Drawing for the job (mm, zero at the part's lowest x, y, z). Give positions to 0.01 mm unless a question says otherwise; leave off trailing zeros. Write each loop counter-clockwise with the first axis right and the second up, starting at its lowest first coordinate (ties: lowest second). Pieces come first, ordered by that corner, then holes.
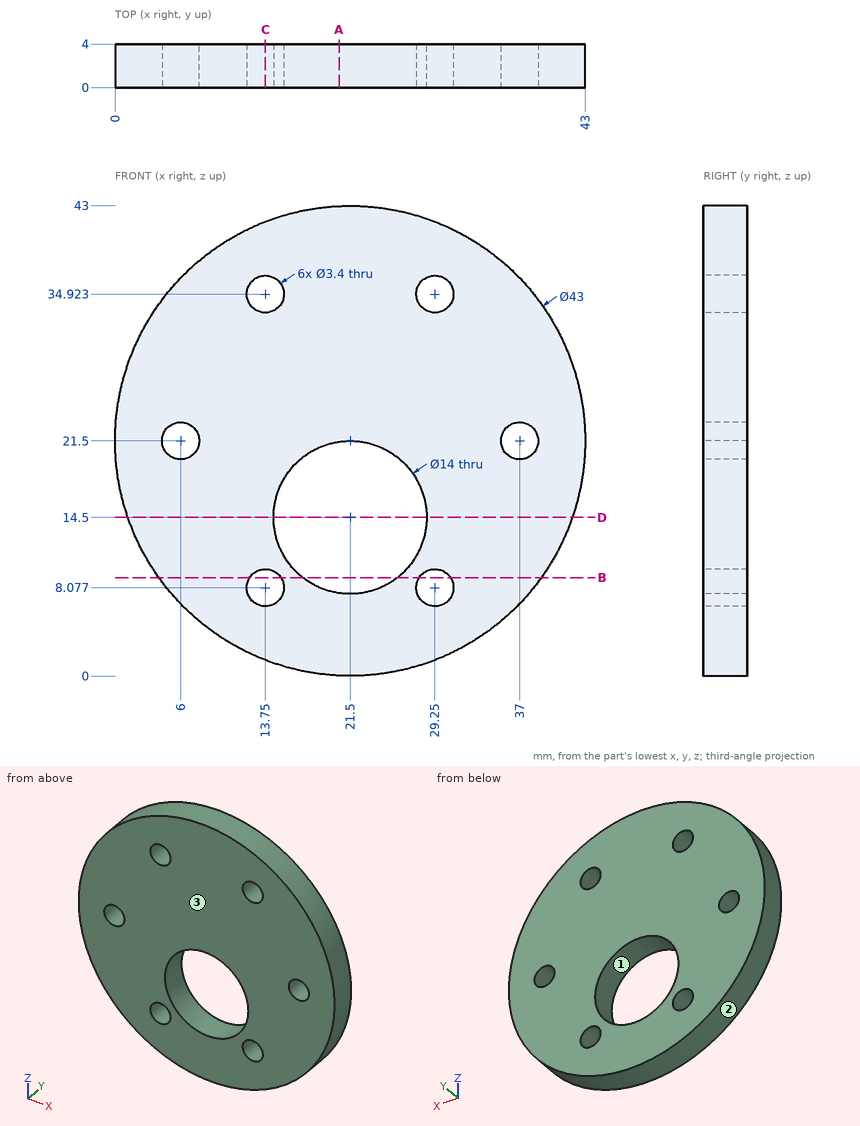
1. Pull direction X, two halves, no side cores. Call the marked faces 1, 2 and 3: +X half, -X half, draft (parallel to the pull), parting line (faces both ways), or undercut.
Calculated:
face 1: undercut
face 2: parting line
face 3: draft
2. Probe probe 1 along X at (y, z) = (2.4, 20.5) (1 decimal); probe 2 along Z at (x, y) = (21.5, 3.05); probe 3 along Z at (x, y) = (13.75, 2.45) (1 decimal). List the from-to ranges inside material, lowest first.
Calculated:
probe 1: x = 0 to 4.6, 7.4 to 17.9, 25.1 to 35.6, 38.4 to 43
probe 2: z = 0 to 7.5, 21.5 to 43
probe 3: z = 1.4 to 6.4, 9.8 to 33.2, 36.6 to 41.6
3. Slice it at A-A, the plane x = 20.5. Write the cut outline in (y, z), and give its area (3 significant figures).
Calculated:
outline: (0, 0.02) - (4, 0.02) - (4, 7.57) - (0, 7.57) - close; (0, 21.43) - (4, 21.43) - (4, 42.98) - (0, 42.98) - close
area: 116 mm2
4. Slice it at C-C, the plane x = 13.75. Write the cut outline in (y, z) (1 decimal).
Calculated:
outline: (0, 1.4) - (4, 1.4) - (4, 6.4) - (0, 6.4) - close; (0, 9.8) - (4, 9.8) - (4, 33.2) - (0, 33.2) - close; (0, 36.6) - (4, 36.6) - (4, 41.6) - (0, 41.6) - close
5. Pin check, flat tips, straight feed: P1, Ø4, axis at x = 6, z = 21.5, coming from the -Y side; P2, Ø3, axis at x = 13.75, z = 8.08, coming from the +Y side; P3, Ø2, axis at x = 11, y = 2.5, coming from the -Z side; P4, Ø2, axis at x = 31, y = 0.5, coming from the -Z side. Stop position of each tip, or through.
Calculated:
P1: stops at y = 0
P2: passes through
P3: stops at z = 2.21
P4: stops at z = 1.75
6. Slice it at B-B, the plane z = 9. Write the cut outline in (x, y).
Calculated:
outline: (4.01, 0) - (12.32, 0) - (12.32, 4) - (4.01, 4) - close; (15.18, 0) - (17.17, 0) - (17.17, 4) - (15.18, 4) - close; (25.83, 0) - (27.82, 0) - (27.82, 4) - (25.83, 4) - close; (30.68, 0) - (38.99, 0) - (38.99, 4) - (30.68, 4) - close
7. Slice it at D-D, the plane z = 14.5. Write the cut outline in (x, y), and give its area (3 significant figures).
Calculated:
outline: (1.17, 0) - (14.5, 0) - (14.5, 4) - (1.17, 4) - close; (28.5, 0) - (41.83, 0) - (41.83, 4) - (28.5, 4) - close
area: 107 mm2
